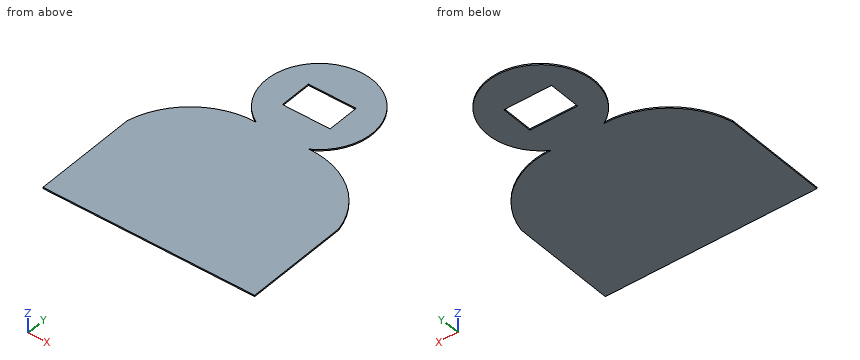
from build123d import *

# Parameters (mm, degrees)
SKETCH1_W           = 180
SKETCH1_H           = 122
BOSS_EXTRUDE1_DEPTH = 5


with BuildPart() as part:
    # Sketch1 → Boss-Extrude1 (new body)
    with BuildSketch(Plane.XY):
        with BuildLine():
            Line((-447.591580819, 337.042460879), (-447.591580819, -59.082484796))
            Line((-447.591580819, -59.082484796), (352.408419181, -59.082484796))
            Line((352.408419181, -59.082484796), (352.408419181, 337.042460879))
            ThreePointArc((352.408419181, 337.042460879), (243.83842934, 506.739072759), (52.408419181, 569.5))
            ThreePointArc((52.408419181, 569.5), (-47.591580819, 942.705080757), (-147.591580819, 569.5))
            ThreePointArc((-147.591580819, 569.5), (-339.021590977, 506.739072759), (-447.591580819, 337.042460879))
        make_face()
        with Locations((-47.591580819, 742.705080757)):
            Rectangle(SKETCH1_W, SKETCH1_H, mode=Mode.SUBTRACT)
    extrude(amount=BOSS_EXTRUDE1_DEPTH)


solid = part.part
Here's how the part is built. I have some questions about the finished solid (model axes, mm). Round coordinates to 2 decimals unless told otherwise and drop trailing zeros. Write each loop counter-clockwise with the first axis right and the second up, starting at its lowest first coordinate (ties: lowest second). Pieces come first, ordered by that corner, then holes.
1. Suppose I cut it at D-D (y = 499.5). List the corners of the cut face in (x, z) for me.
2. I need wall thicknesses on L1, parallel to X at y = 742, z = 2.15; L2, parallel to Y at x = -117, z = 4.5 (3 decimals); L3, parallel to Y at x = -153.5, z = 4.65. Which ranges of each line are inside material? Lowest first, please.
3. Suppose I cut it at A-A (z = 3.1). List the corners of the cut face in (x, y) for me.
4. Suppose I cut it at C-C (y = 713). List the corners of the cut face in (x, z) for me.
5. Suppose I cut it at B-B (x = -29.5). List the corners of the cut face in (y, z) for me.
6. Will these pins go through, and if not, where does the flat tip stop? pin 1 Ø2.5 at (y, z) = (733, 1.5) entering from +X; pin 2 Ø1.5 at (y, z) = (447.5, 3.5) entering from -X; pin 3 Ø3 at (x, z) = (-112.5, 3.5) entering from +Y.
Answer sheet:
1. outline: (-348, 0) - (252.82, 0) - (252.82, 5) - (-348, 5) - close
2. L1: x = -247.59 to -137.59, 42.41 to 152.41
2. L2: y = -59.082 to 681.705, 803.705 to 930.275
2. L3: y = -59.08 to 569.59, 573.05 to 912.36
3. outline: (-447.59, -59.08) - (352.41, -59.08) - (352.41, 337.04) arc R300 ccw to (52.41, 569.5) arc R200 ccw (long way) to (-147.59, 569.5) arc R300 ccw to (-447.59, 337.04) - close; hole (-137.59, 681.71) - (42.41, 681.71) - (42.41, 803.71) - (-137.59, 803.71) - close
4. outline: (-245.37, 0) - (-137.59, 0) - (-137.59, 5) - (-245.37, 5) - close; (42.41, 0) - (150.19, 0) - (150.19, 5) - (42.41, 5) - close
5. outline: (-59.08, 0) - (681.71, 0) - (681.71, 5) - (-59.08, 5) - close; (803.71, 0) - (941.89, 0) - (941.89, 5) - (803.71, 5) - close
6. pin 1: stops at x = 152.23
6. pin 2: stops at x = -397.38
6. pin 3: stops at y = 932.39
